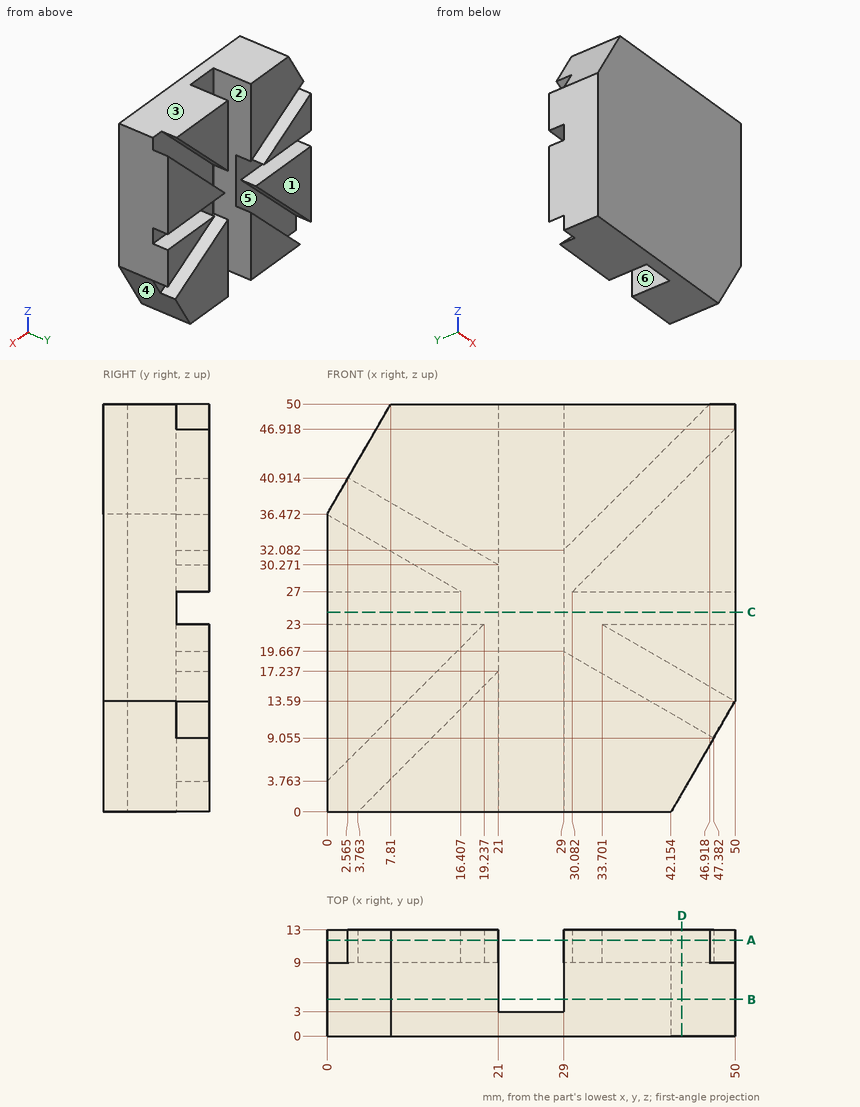
Print and shaded views of the part. All mm, measured from the part's lowest x, y and z. A direction names the side the tool comes from. Coordinates: 2 decimals unless noted, no trailing zeros. Order: outer loops, then holes, each group sorted by start corner. A loop starts at its lowest first (then second) coordinate and runs counter-clockwise, first axis right, second up. Notation, with made-up numbers: M 82,68.5 L 91,68.5 A24 ccw 91,102.5 Z; hole C -27,30 d5. An arc over 180 degrees is marked long. One line per question, with ' | ' between items. Start each with the question number.
Q1. 3-axis set-ups, long thin cutter, end or side, ignore diameter. For the marked faces 1 and 2: which of +Z, -Z, +X, -X, +Y, -Y reach the whole face in a straight line?
Q2. Saw through at B-B (y = 4.5). List the corners of the cut face in (x, z) (1 decimal), then the cut area to 3 significant figures.
Q3. Probe L1, parallel to X at y = 3.75, z = 24; L2, parallel to Z at x = 6, y = 9.5 (1 decimal); L3, parallel to Z at x = 34.5, y = 10.75. List the from-to ranges inside material, lowest first. Write a range as from..to.
Q4. Saw through at C-C (z = 24.5). List the corners of the cut face in (x, y), then the cut area to 3 significant figures.
Q5. Flat gauge pins, fed straight in: pin 1 Ø2 at (x, y) = (43.5, 11.5) entering from -Z; pin 2 Ø1.5 at (x, z) = (24, 29.5) entering from +Y. Where does each tip first touch, or does it go through?
Q6. Saw through at D-D (x = 43.5). List the corners of the cut face in (y, z) (1 decimal), then the cut area to 3 significant figures.
Q7. Saw through at A-A (y = 11.75). List the corners of the cut face in (x, z) (1 decimal), then the cut area to 3 significant figures.
Q8. Two-plate mould, pull along Z, no slides. Class the marked faces 3, 4, 5 and 6: +Z half, -Z half, draft (parallel to the pull), parting line (faces both ways), or undercut.
Check values:
1) face 1: +Z, -Z, +X, -X, +Y | face 2: +Z, -Z, +Y
2) outline: M 0,0 L 21,0 L 21,50 L 7.8,50 L 0,36.5 Z; M 29,0 L 42.2,0 L 50,13.6 L 50,50 L 29,50 Z | area: 1,990 mm2
3) L1: x = 0..21, 29..50 | L2: z = 0..2.2, 9.8..23, 27..33, 38.9..46.9 | L3: z = 0..16.49, 22.54..23, 27..31.42, 37.58..50
4) outline: M 0,0 L 50,0 L 50,9 L 29,9 L 29,3 L 21,3 L 21,9 L 0,9 Z | area: 402 mm2
5) pin 1: stops at z = 0.6 | pin 2: stops at y = 3
6) outline: M 0,2.3 L 13,2.3 L 13,11.3 L 9,11.3 L 9,17.3 L 13,17.3 L 13,23 L 9,23 L 9,27 L 13,27 L 13,40.4 L 9,40.4 L 9,46.6 L 13,46.6 L 13,50 L 0,50 Z | area: 555 mm2
7) outline: M 0,3.8 L 19.2,23 L 0,23 Z; M 0,27 L 16.4,27 L 0,36.5 Z; M 2.6,40.9 L 21,30.3 L 21,50 L 7.8,50 Z; M 3.8,0 L 21,0 L 21,17.2 Z; M 29,0 L 42.2,0 L 47.4,9.1 L 29,19.7 Z; M 29,32.1 L 46.9,50 L 29,50 Z; M 30.1,27 L 50,27 L 50,46.9 Z; M 33.7,23 L 50,13.6 L 50,23 Z | area: 1,330 mm2
8) face 3: +Z half | face 4: -Z half | face 5: undercut | face 6: draft
